CAD build for the part. Positions are in the model's coordinates, mm. Face numbers are marked on the shaded views. A direction names the side the tool comes from. Round coordinates to 2 decimals unless told otherwise and drop trailing zeros. Write each loop counter-clockwise with the first axis right and the second up, starting at its lowest first coordinate (ties: lowest second). Pieces come first, ordered by that corner, then holes. Notation, with made-up numbers: (89, 78) -> (100, 78) arc R33 ccw to (100, 116) -> close; hole circle Ø7 at (-12, 84.5). An arc over 180 degrees is marked (long way). Put each result on its own line as item: value. Start each with the question number.
1. Saw through at C-C on x = 0. List the corners of the cut face in (y, z) (3 decimals), and give its area (3 significant figures).
2. 3-axis set-ups, long thin cutter, end or side, ignore diameter. For the marked faces 4 and 5: which of +Z, -Z, +X, -X, +Y, -Y reach the whole face in a straight line?
3. Flat gauge pins, fed straight in: P1, Ø3.5, axis at x = 3.315, z = 16.74, coming from the +Y side; P2, Ø3, axis at y = 1.5, z = 16.5, coming from the +X side; P3, Ø1.5, axis at x = -1, z = 14.5, coming from the -Y side. Where does each tip first touch, or does it go through?
4. Saw through at B-B on z = 16.74. List the corners of the cut face in (x, y) (3 decimals).
5. Pull direction Z, two halves, no side cores. Call the marked faces 1, 2 and 3: pulls with the +Z half, pulls with the -Z half, needs draft (parallel to the pull), parting line crosses it, or undercut.
6. Saw through at D-D on y = 1.75. List the corners of the cut face in (x, z) (3 decimals).
7. Saw through at A-A on z = 0. List the corners of the cut face in (x, y) (3 decimals).
8. Drill centre lines: line 1 (X direction, y = 1.8, z = 16.74) (3 decimals); line 2 (X direction, y = -0.25, z = 0) (3 decimals); line 3 (Y direction, x = -7.75, z = 4). Where is each one in solid material? Low to high. Write a range as from..to.
from build123d import *

# Parameters (mm, degrees)
BOSS_EXTRUDE1_DEPTH = 2.83
BOSS_EXTRUDE2_START = 4.48
SKETCH2_R           = 12.05
BOSS_EXTRUDE2_DEPTH = 4.48
SKETCH3_R           = 6.34
BOSS_EXTRUDE3_DEPTH = 2.27
SKETCH4_R           = 3.035
CUT_EXTRUDE1_DEPTH  = 29.151799232
SKETCH5_R           = 1.53
CUT_EXTRUDE2_DEPTH  = 28.46240157


with BuildPart() as part:
    # Sketch1 → Boss-Extrude1 (new body)
    with BuildSketch(Plane(origin=(0, 0, 0), x_dir=(1, 0, 0), z_dir=(0, 1, 0))):
        with BuildLine():
            Line((-6.55, -23.57), (6.55, -23.57))
            ThreePointArc((6.55, -23.57), (9.378427125, -22.398427125), (10.55, -19.57))
            Line((10.55, -19.57), (10.55, -14.674703952))
            ThreePointArc((10.55, -14.674703952), (9.86662479, -12.438635975), (8.05, -10.966604709))
            Line((8.05, -10.966604709), (8.05, -8.966604709))
            ThreePointArc((8.05, -8.966604709), (0, 12.05), (-8.05, -8.966604709))
            Line((-8.05, -8.966604709), (-8.05, -10.966604709))
            ThreePointArc((-8.05, -10.966604709), (-9.86662479, -12.438635975), (-10.55, -14.674703952))
            Line((-10.55, -14.674703952), (-10.55, -19.57))
            ThreePointArc((-10.55, -19.57), (-9.378427125, -22.398427125), (-6.55, -23.57))
        make_face()
    extrude(amount=BOSS_EXTRUDE1_DEPTH)

    # Sketch2 → Boss-Extrude2 (add)
    with BuildSketch(Plane.XZ.offset(BOSS_EXTRUDE2_START)):
        with Locations(Location((0, 0, 0), (0, 0, 270))):
            Circle(SKETCH2_R)
    extrude(amount=-BOSS_EXTRUDE2_DEPTH)

    # Sketch3 → Boss-Extrude3 (add)
    with BuildSketch(Plane(origin=(0, 2.83, 0), x_dir=(1, 0, 0), z_dir=(0, 1, 0))):
        with Locations(Location((0, 0, 0), (0, 0, 90))):
            Circle(SKETCH3_R)
    extrude(amount=BOSS_EXTRUDE3_DEPTH)

    # Sketch4 → Cut-Extrude1 (cut, through all)
    with BuildSketch(Plane(origin=(0, 5.1, 0), x_dir=(1, 0, 0), z_dir=(0, 1, 0))):
        with Locations(Location((0, 0, 0), (0, 0, 270))):
            Circle(SKETCH4_R)
    extrude(amount=-CUT_EXTRUDE1_DEPTH, mode=Mode.SUBTRACT)

    # Sketch5 → Cut-Extrude2 (cut, through all)
    with BuildSketch(Plane(origin=(0, 2.83, 0), x_dir=(1, 0, 0), z_dir=(0, 1, 0))):
        with Locations(Location((-3.315, -16.74, 0), (0, 0, 270))):
            Circle(SKETCH5_R)
        with Locations(Location((3.315, -16.74, 0), (0, 0, 270))):
            Circle(SKETCH5_R)
    extrude(amount=-CUT_EXTRUDE2_DEPTH, mode=Mode.SUBTRACT)


solid = part.part
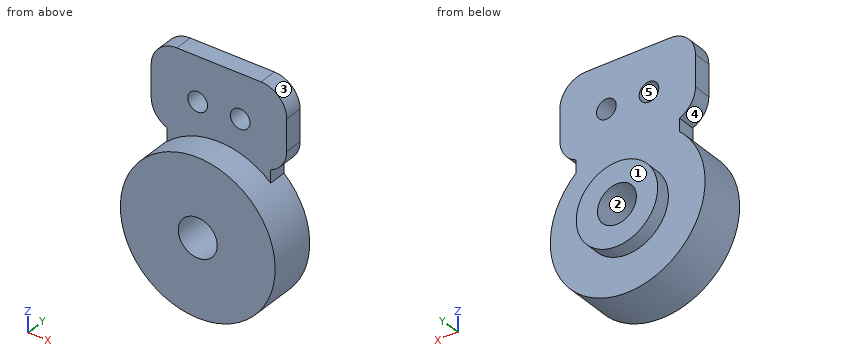
Return value:
1. outline: (-4.48, -12.05) -> (2.83, -12.05) -> (2.83, -6.34) -> (5.1, -6.34) -> (5.1, -3.035) -> (-4.48, -3.035) -> close; (-4.48, 3.035) -> (5.1, 3.035) -> (5.1, 6.34) -> (2.83, 6.34) -> (2.83, 23.57) -> (0, 23.57) -> (0, 12.05) -> (-4.48, 12.05) -> close
1. area: 179 mm^2
2. face 4: -X, +Y, -Y
2. face 5: +Y, -Y
3. P1: stops at y = 2.83
3. P2: stops at x = 10.55
3. P3: stops at y = 0
4. outline: (-10.55, 0) -> (-4.845, 0) -> (-4.845, 2.83) -> (-10.55, 2.83) -> close; (-1.785, 0) -> (1.785, 0) -> (1.785, 2.83) -> (-1.785, 2.83) -> close; (4.845, 0) -> (10.55, 0) -> (10.55, 2.83) -> (4.845, 2.83) -> close
5. face 1: needs draft
5. face 2: undercut
5. face 3: pulls with the +Z half
6. outline: (-10.55, 14.675) arc R4 ccw to (-8.05, 10.967) -> (-8.05, 8.967) arc R12.05 ccw (long way) to (8.05, 8.967) -> (8.05, 10.967) arc R4 ccw to (10.55, 14.675) -> (10.55, 19.57) arc R4 ccw to (6.55, 23.57) -> (-6.55, 23.57) arc R4 ccw to (-10.55, 19.57) -> close; hole circle Ø3.06 at (-3.315, 16.74); hole circle Ø6.07 at (0, 0); hole circle Ø3.06 at (3.315, 16.74)
7. outline: (-12.05, -4.48) -> (-3.035, -4.48) -> (-3.035, 5.1) -> (-6.34, 5.1) -> (-6.34, 2.83) -> (-12.05, 2.83) -> close; (3.035, -4.48) -> (12.05, -4.48) -> (12.05, 2.83) -> (6.34, 2.83) -> (6.34, 5.1) -> (3.035, 5.1) -> close
8. line 1: x = -10.55..-4.845, -1.785..1.785, 4.845..10.55
8. line 2: x = -12.05..-3.035, 3.035..12.05
8. line 3: y = -4.48..2.83
